```python
from build123d import *

# Parameters (mm, degrees)
F0_W     = 25.4
F0_H     = 50.8
F1_DEPTH = 177.8
F2_R     = 12.7
F3_DEPTH = 38.1
F5_R     = 50.8
F7_D     = 50.8
F8_R     = 50.8


with BuildPart() as f1:
    # F0 (on Right) → F1 (new body)
    with BuildSketch(Plane.YZ):
        with BuildLine():
            ThreePointArc((12.7, -35.9210244843), (31.1085197333, -21.9970452561), (38.1, 0))
            ThreePointArc((38.1, 0), (31.1085197333, 21.9970452561), (12.7, 35.9210244843))
            Line((12.7, 35.9210244843), (12.7, -35.9210244843))
        make_face()
        with BuildLine():
            Line((12.7, -35.9210244843), (12.7, 35.9210244843))
            ThreePointArc((12.7, 35.9210244843), (0, 38.1), (-12.7, 35.9210244843))
            Line((-12.7, 35.9210244843), (-12.7, -35.9210244843))
            ThreePointArc((-12.7, -35.9210244843), (0, -38.1), (12.7, -35.9210244843))
        make_face()
        with BuildLine():
            ThreePointArc((-12.7, 35.9210244843), (0, 38.1), (12.7, 35.9210244843))
            Line((12.7, 35.9210244843), (12.7, 127))
            Line((12.7, 127), (-12.7, 127))
            Line((-12.7, 127), (-12.7, 35.9210244843))
        make_face()
        with BuildLine():
            Line((12.7, -127), (12.7, -35.9210244843))
            ThreePointArc((12.7, -35.9210244843), (0, -38.1), (-12.7, -35.9210244843))
            Line((-12.7, -35.9210244843), (-12.7, -127))
            Line((-12.7, -127), (12.7, -127))
        make_face()
        with BuildLine():
            Line((-12.7, -35.9210244843), (-12.7, 35.9210244843))
            ThreePointArc((-12.7, 35.9210244843), (-38.1, 0), (-12.7, -35.9210244843))
        make_face()
        with Locations((0, -152.4)):
            Rectangle(F0_W, F0_H)
    extrude(amount=F1_DEPTH)

    # F2 (on face) → F3 (join)
    with BuildSketch(Plane(origin=(0, 12.7, 0), x_dir=(-1, 0, 0), z_dir=(0, 1, 0))):
        with Locations((-152.4, 88.9)):
            Circle(F2_R)
        with Locations((-25.4, 88.9)):
            Circle(F2_R)
        with Locations((-25.4, -114.3)):
            Circle(F2_R)
        with Locations((-152.4, -114.3)):
            Circle(F2_R)
    extrude(amount=F3_DEPTH)

    # F4: F1 across plane


with BuildPart() as f1_1:
    add(f1.part)
    add(f1.part.mirror(Plane.XZ))

    # F5
    f5_edges = [f1_1.edges().sort_by_distance(p)[0] for p in [
        (177.8, 0, 127),
        (0, 0, 127),
    ]]
    fillet(f5_edges, radius=F5_R)

    # F7 (through all)
    with Locations(Plane(origin=(0, 12.7, 0), x_dir=(-1, 0, 0), z_dir=(0, 1, 0))):
        with Locations((-88.9, -127)):
            Hole(F7_D / 2)

    # F8
    f8_edges = [f1_1.edges().sort_by_distance(p)[0] for p in [
        (177.8, 0, -177.8),
        (0, 0, -177.8),
    ]]
    fillet(f8_edges, radius=F8_R)


solid = f1_1.part
```
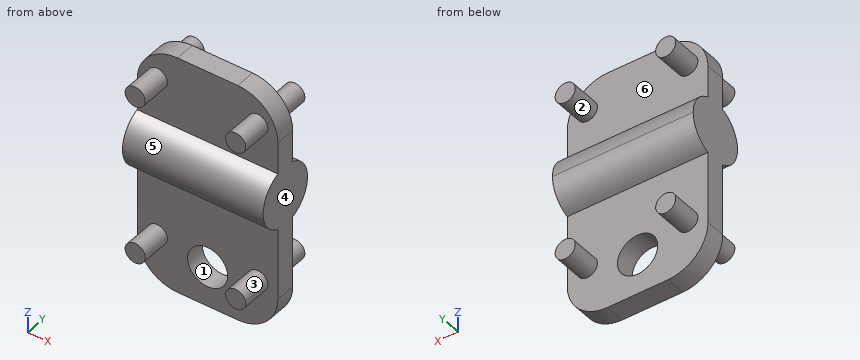
Check sheet for the modelled part. Datum: model origin and axes. Units: mm. Face numbers are marked on the shaded views. A direction names the side the tool comes from. Round coordinates to 2 decimals unless told otherwise and drop trailing zeros. Loops run counter-clockwise (first coordinate to the right, second up) from the corner with the lowest first, then second, coordinate; pieces in that order, holes last. Notation, with made-up numbers: (80, 78) -> (124, 78) arc R31 cw to (124, 110) -> close; hole circle Ø1 at (8, 78.25). An arc over 180 degrees is marked (long way). Write item = value, one per line. Start each with the question number.
1) Sectioned sample at C-C, the plane y = 2. Record the cut outline in (x, z), plus the area to 3 significant figures.
2) Sectioned sample at D-D, the plane y = -25.5. Record the cut outline in (x, z).
3) Release check for a two-part mould opening along X. For the marked faces 4, 5 and 6 record: released by +X, released by -X, zero draft, split by the parting line, or undercut.
4) Set-up check for the marked faces 1, 2 and 3: record each of +Z, -Z, +X, -X, +Y, -Y from which the full face is reachable in a straight line by a thin tool's end or side.
5) Thickness scan on probe 1 along Z at (x, y) = (88.9, 6.5); probe 2 along Z at (x, y) = (142, -29.5); probe 3 along Y at (x, z) = (26, 54). Record the ranges inside material, lowest first.
6) Sectioned sample at A-A, the plane x = 88.9. Record the cut outline in (y, z), plus the area to 3 significant figures.
7) Sectioned sample at B-B, the plane z = -114.3. Record the cut outline in (x, y).
8) Gauge pin test, flat ends, axial feed: pin 1 Ø12 at (x, z) = (110.5, -57) entering from -Y; pin 2 Ø5 at (x, y) = (18, -0.5) entering from -Z; pin 3 Ø1 at (y, z) = (27.5, -111) entering from +X. Record the tip position at first contact, or that the pin passes through.
Results are:
q1.outline = (0, -127) arc R50.8 ccw to (50.8, -177.8) -> (127, -177.8) arc R50.8 ccw to (177.8, -127) -> (177.8, 76.2) arc R50.8 ccw to (127, 127) -> (50.8, 127) arc R50.8 ccw to (0, 76.2) -> close; hole circle Ø50.8 at (88.9, -127)
q1.area = 50,000 mm^2
q2.outline = (0, -28.31) -> (177.8, -28.31) -> (177.8, 28.31) -> (0, 28.31) -> close; circle Ø25.4 at (25.4, -114.3); circle Ø25.4 at (25.4, 88.9); circle Ø25.4 at (152.4, -114.3); circle Ø25.4 at (152.4, 88.9)
q3.face_4 = released by +X
q3.face_5 = zero draft
q3.face_6 = undercut
q4.face_1 = +Y, -Y
q4.face_2 = +Y
q4.face_3 = -Y
q5.probe_1 = -177.8 to -152.4, -101.6 to 127
q5.probe_2 = -121.59 to -107.01, -24.11 to 24.11, 81.61 to 96.19
q5.probe_3 = -12.7 to 12.7
q6.outline = (-12.7, -177.8) -> (12.7, -177.8) -> (12.7, -152.4) -> (-12.7, -152.4) -> close; (-12.7, -101.6) -> (12.7, -101.6) -> (12.7, -35.92) arc R38.1 ccw to (12.7, 35.92) -> (12.7, 127) -> (-12.7, 127) -> (-12.7, 35.92) arc R38.1 ccw to (-12.7, -35.92) -> close
q6.area = 9,110 mm^2
q7.outline = (0, -12.7) -> (12.7, -12.7) -> (12.7, -50.8) -> (38.1, -50.8) -> (38.1, -12.7) -> (66.9, -12.7) -> (66.9, 12.7) -> (38.1, 12.7) -> (38.1, 50.8) -> (12.7, 50.8) -> (12.7, 12.7) -> (0, 12.7) -> close; (110.9, -12.7) -> (139.7, -12.7) -> (139.7, -50.8) -> (165.1, -50.8) -> (165.1, -12.7) -> (177.8, -12.7) -> (177.8, 12.7) -> (165.1, 12.7) -> (165.1, 50.8) -> (139.7, 50.8) -> (139.7, 12.7) -> (110.9, 12.7) -> close
q8.pin_1 = -12.7
q8.pin_2 = -167.77
q8.pin_3 = 164.79
